from build123d import *

# Parameters (mm, degrees)
F2_DEPTH = 63.5010001
F3_R     = 5.08
F5_R     = 5.08
F6_R     = 5.08


# Not quite as in the source:
# - a fillet or chamfer that OpenCascade refuses, or shapes differently, is made with other operations: its cross-section is extruded or revolved along the edge and cut away or added


with BuildPart() as f1:
    # F0 (on Front) → F1 (revolve)
    with BuildSketch(Plane.XZ):
        with BuildLine():
            ThreePointArc((4.5341940657, 59.2838630326), (2.9433454488, 62.1191947856), (0, 63.5))
            Line((0, 63.5), (0, 0))
            Line((0, 0), (2.5480911136, 0))
            Line((2.5480911136, 0), (6.6250329837, 10.4471649975))
            Line((6.6250329837, 10.4471649975), (10.9556252941, 16.1543861032))
            Line((10.9556252941, 16.1543861032), (30.48, 16.1543861032))
            Line((30.48, 16.1543861032), (30.4299078499, 21.4240159839))
            Line((30.4299078499, 21.4240159839), (20.699405237, 21.4240159839))
            ThreePointArc((20.699405237, 21.4240159839), (16.6336106625, 21.5337881018), (12.597086859, 22.0329985023))
            ThreePointArc((12.597086859, 22.0329985023), (4.6942529553, 39.8204748482), (4.5341940657, 59.2838630326))
        make_face()
    revolve(axis=Axis((0, 0, 31.75), (0, 0, -1)))

    # F2 (cut, through all): a face of the model
    f2_faces = [f1.faces().sort_by_distance(p)[0] for p in [
        (0, 0, 0),
    ]]
    extrude(f2_faces, amount=-F2_DEPTH, mode=Mode.SUBTRACT)

    # F3
    f3_edges = [f1.edges().sort_by_distance(p)[0] for p in [
        (-10.955625, 0, 16.154386),
        (-30.48, 0, 16.154386),
    ]]
    fillet(f3_edges, radius=F3_R)

    # F4: chamfer of 5.08 on 1 edges, made by hand

    # F4_s1 → F4_t2 (revolve, cut)
    with BuildSketch(Plane.XZ):
        Polygon((30.478195231, 16.3442454843), (25.3499078499, 21.4240159839), (30.4299078499, 21.4240159839), align=None)
    revolve(axis=Axis((0, 0, 21.4240159839), (0, 0, -1)), mode=Mode.SUBTRACT)

    # F5
    f5_edges = [f1.edges().sort_by_distance(p)[0] for p in [
        (-20.699405, 0, 21.424016),
        (-12.597087, 0, 22.032999),
        (16.633611, 0, 21.533788),
    ]]
    fillet(f5_edges, radius=F5_R)

    # F6
    f6_edges = [f1.edges().sort_by_distance(p)[0] for p in [
        (-25.349908, 0, 21.424016),
        (-20.699405, 0, 21.424016),
    ]]
    fillet(f6_edges, radius=F6_R)


solid = f1.part
Here's how the part is built. I have some questions about the finished solid (model axes, mm). Coordinates: 2 decimals unless noted, no trailing zeros. Order: outer loops, then holes, each group sorted by start corner. A loop starts at its lowest first (then second) coordinate and runs counter-clockwise, first axis right, second up. Notation, with made-up numbers: (56, -19.5) -> (84, -19.5) arc R26 ccw to (84, 12.5) -> close; hole circle Ø2 at (85.25, -5). An arc over 180 degrees is marked (long way). Answer in a Markdown table with one row per item.
(1) Will these pins go through, and if not, where does the flat tip stop? pin 1 Ø2 at (x, y) = (18.5, 13) entering from -Z; pin 2 Ø5 at (x, z) = (-1.5, 34) entering from -Y; pin 3 Ø10 at (y, z) = (9.5, 24) entering from -X.
Answer key:
| item | result |
|---|---|
| pin 1 | z = 16.15 |
| pin 2 | y = -7.22 |
| pin 3 | x = -26.38 |
(2) Thinking about a two-plate mould opening in Y: for faces 1 (the face through (25.698, -8.093, 19.846)), 2 (the face through (-16, 14, 21.424)), 3 (the face through (-2.546, -0.112, 30.789)), which applies, +Y half, -Y half, draft (parallel to the pull), parting line (faces both ways), or undercut?
Answer key:
| item | result |
|---|---|
| face 1 | parting line |
| face 2 | draft |
| face 3 | undercut |
(3) I want a section at B-B on z = 51.5. List the corners of the cut face in (x, y) for me.
Answer key:
| item | result |
|---|---|
| outline | circle Ø7.27 at (0, 0); hole circle Ø5.1 at (0, 0) |
(4) Please list where these lines run through material, in increasing order: probe 1 along Y at (x, z) = (0, 26.5); probe 2 along Y at (x, z) = (0, 24); probe 3 along X at (y, z) = (0, 29).
Answer key:
| item | result |
|---|---|
| probe 1 | -9.75 to -2.55, 2.55 to 9.75 |
| probe 2 | -11.26 to -2.55, 2.55 to 11.26 |
| probe 3 | -8.44 to -2.55, 2.55 to 8.44 |
(5) I want a section at A-A on z = 43.5. List the corners of the cut face in (x, y) for me, then the cut area to 3 significant figures.
Answer key:
| item | result |
|---|---|
| outline | circle Ø8.09 at (0, 0); hole circle Ø5.1 at (0, 0) |
| area | 31.1 mm^2 |
